```python
from build123d import *

# Parameters (mm, degrees)
F0_W      = 300
F0_H      = 25
F1_DEPTH  = 4
F2_W      = 300
F2_H      = 5
F3_DEPTH  = 60
F4_SIZE2  = 55.980762
F4_SIZE   = 15
F5_SIZE   = 2
F6_W      = 50
F6_H      = 20
F7_DEPTH  = 8
F9_R      = 2.5
F10_DEPTH = 5
F11_R     = 2.5
F12_DEPTH = 5
F13_W     = 35
F13_H     = 25
F14_DEPTH = 8
F15_R     = 2.5
F16_DEPTH = 35


with BuildPart() as f1:
    # F0 (on Top) → F1 (new body)
    with BuildSketch(Plane.XY):
        Rectangle(F0_W, F0_H)
    extrude(amount=F1_DEPTH)

    # F2 (on face) → F3 (join)
    with BuildSketch(Plane.XY.offset(4)):
        with Locations((0, -10)):
            Rectangle(F2_W, F2_H)
    extrude(amount=F3_DEPTH)

    # F4
    f4_edges = [f1.edges().sort_by_distance(p)[0] for p in [
        (-150, -10, 64),
        (150, -10, 64),
    ]]
    chamfer(f4_edges, length=F4_SIZE, length2=F4_SIZE2)

    # F5
    f5_edges = [f1.edges().sort_by_distance(p)[0] for p in [
        (0, 12.5, 4),
    ]]
    chamfer(f5_edges, length=F5_SIZE)

    # F6 (on face) → F7 (join)
    with BuildSketch(Plane.XZ.offset(12.5)):
        with Locations((0, 64)):
            Rectangle(F6_W, F6_H)
    extrude(amount=F7_DEPTH)

    # F9 (on face) → F10 (join)
    with BuildSketch(Plane(origin=(-25, 0, 0), x_dir=(0, -1, 0), z_dir=(-1, 0, 0))):
        with Locations((17.5, 69)):
            Circle(F9_R)
        with Locations((17.5, 59)):
            Circle(F9_R)
    extrude(amount=F10_DEPTH)

    # F11 (on face) → F12 (join)
    with BuildSketch(Plane.YZ.offset(25)):
        with Locations((-17.5, 59)):
            Circle(F11_R)
        with Locations((-17.5, 69)):
            Circle(F11_R)
    extrude(amount=F12_DEPTH)

    # F13 (on face) → F14 (cut)
    with BuildSketch(Plane.XZ.offset(20.5)):
        with Locations((0, 73.5)):
            Rectangle(F13_W, F13_H)
    extrude(amount=-F14_DEPTH, mode=Mode.SUBTRACT)

    # F15 (on face) → F16 (join, through all)
    with BuildSketch(Plane(origin=(17.5, 0, 0), x_dir=(0, -1, 0), z_dir=(-1, 0, 0))):
        with Locations((17.5, 69)):
            Circle(F15_R)
    extrude(amount=F16_DEPTH)


solid = f1.part
```
Geometry check sheet. Reference: the model listing, model coordinates, mm. A direction names the side the tool comes from. Coordinates: 2 decimals unless noted, no trailing zeros. Loops run counter-clockwise (first coordinate to the right, second up) from the corner with the lowest first, then second, coordinate; pieces in that order, holes last. Notation, with made-up numbers: (67.25, -7) - (126.25, -7) arc R17 cw to (126.25, 1) - close; hole circle Ø10 at (-25.5, -24.75). An arc over 180 degrees is marked (long way). One line per item, written item: value. Start each with the question number.
(1) Mould release check, pull along Z, two halves, no side actions. Record for faces 5 (the cylindrical face through (27, -19, 67)), 6 (the flat face through (21, -12.5, 69)), 7 (the flat face through (-2, 2, 4)): released by +Z, released by -Z, zero draft, split by the parting line, or undercut.
(2) Cross-section at A-A on x = -14.5. Enter the section's corners in (y, z).
(3) Cross-section at B-B on y = -17.5. Enter the section's corners in (x, z).
(4) Depth check by flat-ended pin: P1, Ø2.5, axis at y = -17, z = 70, coming from the +X side; P2, Ø4, axis at x = -42.5, y = -14, coming from the +Z side; P3, Ø1.5, axis at x = 69, y = 8, coming from the +Z side; P4, Ø5, axis at y = -3, z = 12, coming from the -X side. Enter the tip coordinate at first touch or a pass-through.
(5) Material ranges on line 1 (Y direction, x = 71, z = 56); line 2 (Z direction, x = -42, y = -5); line 3 (X direction, y = -14, z = 57), recorded low to high. Write a range as [from, to].
(6) Tool access check on faces 1 (the flat face through (30, -18, 59)), 2 (the cylindrical face through (0, -16, 67)), 3 (the flat face through (-1, -10, 64)), 4 (the cylindrical face through (-27, -16, 67)). Record the directions out of +Z, -Z, +X, -X, +Y, -Y that give a thin tool (end or side, any length) a straight path to the whole face; none if there is none.
(7) Cross-section at C-C on x = -80. Enter the section's corners in (y, z), plus the area to 3 significant figures.
(8) Cross-section at D-D on z = 28. Enter the section's corners in (x, y).
Results below:
1. face 5: undercut
1. face 6: zero draft
1. face 7: released by +Z
2. outline: (-20.5, 54) - (-12.5, 54) - (-12.5, 0) - (12.5, 0) - (12.5, 2) - (10.5, 4) - (-7.5, 4) - (-7.5, 64) - (-12.5, 64) - (-12.5, 61) - (-20.5, 61) - close; circle Ø5 at (-17.5, 69)
3. outline: (-30, 56.5) - (-25, 56.5) - (-25, 54) - (25, 54) - (25, 56.5) - (30, 56.5) - (30, 61.5) - (25, 61.5) - (25, 66.5) - (30, 66.5) - (30, 71.5) - (25, 71.5) - (25, 74) - (17.5, 74) - (17.5, 71.5) - (-17.5, 71.5) - (-17.5, 74) - (-25, 74) - (-25, 71.5) - (-30, 71.5) - (-30, 66.5) - (-25, 66.5) - (-25, 61.5) - (-30, 61.5) - close; hole (-17.5, 61) - (17.5, 61) - (17.5, 66.5) - (-17.5, 66.5) - close
4. P1: stops at x = 30
4. P2: stops at z = 64
4. P3: stops at z = 4
4. P4: passes through
5. line 1: y = [-12.5, -7.5]
5. line 2: z = [0, 4]
5. line 3: x = [-25, 25]
6. face 1: +Z, -Z, +X, -Y
6. face 2: none
6. face 3: +Z, +X, -X, +Y
6. face 4: -X
7. outline: (-12.5, 0) - (12.5, 0) - (12.5, 2) - (10.5, 4) - (-7.5, 4) - (-7.5, 64) - (-12.5, 64) - close
7. area: 398 mm2
8. outline: (-150, -12.5) - (150, -12.5) - (150, -7.5) - (-150, -7.5) - close
